The model under review builds one solid part; all positions refer to its coordinate system, in mm. A direction names the side the tool comes from. Give positions to 0.01 mm unless a question says otherwise; leave off trailing zeros. Loops run counter-clockwise (first coordinate to the right, second up) from the corner with the lowest first, then second, coordinate; pieces in that order, holes last. Notation, with made-up numbers: M -14,-32 L -9,-32 A7 ccw -9,-20 Z; hole C -0.75,78.5 d6. An arc over 180 degrees is marked long. Return JSON: item names as keys, results as strings.
```python
from build123d import *

# Parameters (mm, degrees)
F0_W      = 20
F0_H      = 40
F1_DEPTH  = 60
F2_R      = 1.5
F2_R_2    = 10
F3_DEPTH  = 6
F4_R      = 2.25
F5_DEPTH  = 6
F6_R      = 2.25
F7_DEPTH  = 6
F9_R      = 4.5
F9_R_2    = 2.25
F11_DEPTH = 20
F10_R     = 4.5
F10_R_2   = 2.25
F12_DEPTH = 20
F8_R      = 4.5
F8_R_2    = 2.25
F13_DEPTH = 20
F14_DEPTH = 25
F15_DEPTH = 25
F16_DEPTH = 25
F17_DEPTH = 15
F18_DEPTH = 15
F19_DEPTH = 15


with BuildPart() as f1:
    # F0 (on Top) → F1 (new body)
    with BuildSketch(Plane.XY):
        with BuildLine():
            Line((47.3205080757, 53.0098987629), (42.9903810568, 55.5098987629))
            Line((42.9903810568, 55.5098987629), (31.7542648054, 36.0483745358))
            Line((31.7542648054, 36.0483745358), (-31.7542648054, 36.0483745358))
            Line((-31.7542648054, 36.0483745358), (-42.9903810568, 55.5098987629))
            Line((-42.9903810568, 55.5098987629), (-47.3205080757, 53.0098987629))
            Line((-47.3205080757, 53.0098987629), (-17.3205080757, 1.0483745358))
            Line((-17.3205080757, 1.0483745358), (-34.6410161514, -8.9516254642))
            Line((-34.6410161514, -8.9516254642), (-14.6410161514, -43.5926416156))
            ThreePointArc((-14.6410161514, -43.5926416156), (0, -52.0456362318), (14.6410161514, -43.5926416156))
            Line((14.6410161514, -43.5926416156), (34.6410161514, -8.9516254642))
            Line((34.6410161514, -8.9516254642), (17.3205080757, 1.0483745358))
            Line((17.3205080757, 1.0483745358), (47.3205080757, 53.0098987629))
        make_face()
        Polygon((-15, -3.3853821939), (-15, -9.7067520427), (-15, -21.9678594557), (-21.3525872607, -21.9678594557), (-27.8108891325, -10.7817524831), align=None, mode=Mode.SUBTRACT)
        with Locations((0, -18.9516254642)):
            Rectangle(F0_W, F0_H, mode=Mode.SUBTRACT)
        Polygon((15, -21.9678594557), (15, -4.4697315388), (15, -3.3853821939), (27.8108891325, -10.7817524831), (21.3525872607, -21.9678594557), align=None, mode=Mode.SUBTRACT)
        Polygon((28.8675134595, 31.0483745358), (14.4337567297, 6.0483745358), (-14.4337567297, 6.0483745358), (-28.8675134595, 31.0483745358), align=None, mode=Mode.SUBTRACT)
    extrude(amount=F1_DEPTH)

    # F2 (on face) → F3 (cut)
    with BuildSketch(Plane(origin=(0, 36.0483745358, 0), x_dir=(-1, 0, 0), z_dir=(0, 1, 0))):
        with Locations((-15.5, 45.5)):
            Circle(F2_R)
        with Locations((15.5, 45.5)):
            Circle(F2_R)
        with Locations((15.5, 14.5)):
            Circle(F2_R)
        with Locations((-15.5, 14.5)):
            Circle(F2_R)
        with Locations((0, 30)):
            Circle(F2_R_2)
    extrude(amount=-F3_DEPTH, mode=Mode.SUBTRACT)

    # F4 (on face) → F5 (cut)
    with BuildSketch(Plane(origin=(-12.5364215664, -7.237906366, 0), x_dir=(0.5, -0.8660254038, 0), z_dir=(-0.8660254038, -0.5, 0))):
        with Locations((-24.5681730185, 50)):
            Circle(F4_R)
        with Locations((-59.5681730185, 50)):
            Circle(F4_R)
        with Locations((-59.5681730185, 10)):
            Circle(F4_R)
        with Locations((-24.5681730185, 10)):
            Circle(F4_R)
    extrude(amount=-F5_DEPTH, mode=Mode.SUBTRACT)

    # F6 (on face) → F7 (cut)
    with BuildSketch(Plane(origin=(12.5364215664, -7.237906366, 0), x_dir=(0.5, 0.8660254038, 0), z_dir=(0.8660254038, -0.5, 0))):
        with Locations((24.5681730185, 50)):
            Circle(F6_R)
        with Locations((59.5681730185, 50)):
            Circle(F6_R)
        with Locations((59.5681730185, 10)):
            Circle(F6_R)
        with Locations((24.5681730185, 10)):
            Circle(F6_R)
    extrude(amount=-F7_DEPTH, mode=Mode.SUBTRACT)

    # F9 (on face) → F11 (join)
    with BuildSketch(Plane.YZ.offset(-10)):
        with Locations((-28.9516254642, 50)):
            Circle(F9_R)
        with Locations((-28.9516254642, 50)):
            Circle(F9_R_2, mode=Mode.SUBTRACT)
        with Locations((-28.9516254642, 10)):
            Circle(F9_R)
        with Locations((-28.9516254642, 10)):
            Circle(F9_R_2, mode=Mode.SUBTRACT)
    extrude(amount=-F11_DEPTH)

    # F10 (on face) → F12 (join)
    with BuildSketch(Plane(origin=(10, 0, 0), x_dir=(0, -1, 0), z_dir=(-1, 0, 0))):
        with Locations((28.9516254642, 10)):
            Circle(F10_R)
        with Locations((28.9516254642, 10)):
            Circle(F10_R_2, mode=Mode.SUBTRACT)
        with Locations((28.9516254642, 50)):
            Circle(F10_R)
        with Locations((28.9516254642, 50)):
            Circle(F10_R_2, mode=Mode.SUBTRACT)
    extrude(amount=-F12_DEPTH)

    # F8 (on face) → F13 (join)
    with BuildSketch(Plane(origin=(0, -38.9516254642, 0), x_dir=(-1, 0, 0), z_dir=(0, 1, 0))):
        with Locations((0, 50)):
            Circle(F8_R)
        with Locations((0, 50)):
            Circle(F8_R_2, mode=Mode.SUBTRACT)
        with BuildLine():
            ThreePointArc((4.5, 10), (3.1819805153, 13.1819805153), (0, 14.5))
            ThreePointArc((0, 14.5), (-3.1819805153, 6.8180194847), (4.5, 10))
        make_face()
        with BuildLine():
            ThreePointArc((0, 12.25), (1.5909902577, 11.5909902577), (2.25, 10))
            ThreePointArc((2.25, 10), (-1.5909902577, 8.4090097423), (0, 12.25))
        make_face(mode=Mode.SUBTRACT)
    extrude(amount=-F13_DEPTH)

    # F10 (on face) → F14 (cut)
    with BuildSketch(Plane(origin=(10, 0, 0), x_dir=(0, -1, 0), z_dir=(-1, 0, 0))):
        with Locations((28.9516254642, 10)):
            Circle(F10_R_2)
        with Locations((28.9516254642, 50)):
            Circle(F10_R_2)
    extrude(amount=-F14_DEPTH, mode=Mode.SUBTRACT)

    # F9 (on face) → F15 (cut)
    with BuildSketch(Plane.YZ.offset(-10)):
        with Locations((-28.9516254642, 50)):
            Circle(F9_R_2)
        with Locations((-28.9516254642, 10)):
            Circle(F9_R_2)
    extrude(amount=-F15_DEPTH, mode=Mode.SUBTRACT)

    # F8 (on face) → F16 (cut)
    with BuildSketch(Plane(origin=(0, -38.9516254642, 0), x_dir=(-1, 0, 0), z_dir=(0, 1, 0))):
        with Locations((0, 50)):
            Circle(F8_R_2)
        with BuildLine():
            ThreePointArc((0, 12.25), (-1.5909902577, 8.4090097423), (2.25, 10))
            ThreePointArc((2.25, 10), (1.5909902577, 11.5909902577), (0, 12.25))
        make_face()
    extrude(amount=-F16_DEPTH, mode=Mode.SUBTRACT)

    # F17 (cut): faces of the model
    f17_faces = [f1.faces().sort_by_distance(p)[0] for p in [
        (4.3727207794, -58.9516254642, 10),
        (4.3727207794, -58.9516254642, 50),
    ]]
    extrude(f17_faces, amount=-F17_DEPTH, mode=Mode.SUBTRACT)

    # F18 (cut): faces of the model
    f18_faces = [f1.faces().sort_by_distance(p)[0] for p in [
        (30, -24.5789046848, 50),
        (30, -24.5789046848, 10),
    ]]
    extrude(f18_faces, amount=-F18_DEPTH, mode=Mode.SUBTRACT)

    # F19 (cut): faces of the model
    f19_faces = [f1.faces().sort_by_distance(p)[0] for p in [
        (-30, -33.3243462436, 10),
        (-30, -33.3243462436, 50),
    ]]
    extrude(f19_faces, amount=-F19_DEPTH, mode=Mode.SUBTRACT)

    # F22 (on 3pt) → F23 (revolve, cut)
    with BuildSketch(Plane(origin=(-15.0459854695, -0.2184772575, 0), x_dir=(-0.014519104, 0.9998945923, 0), z_dir=(0.9998945923, 0.014519104, 0))):
        Polygon((-3.0741950031, 61.4935897481), (-3.1692667399, 60.0088387728), (31.260818243, 45.5124080181), (31.260818243, 47.0371879637), align=None)
    revolve(axis=Axis((-15.2499175488, 13.8258179605, 52.7606233954), (-0.013381382, 0.9215425078, -0.3880468334)), mode=Mode.SUBTRACT)


solid = f1.part
```
1) Consider section D-D on y = -7.5. Write out the cut boundary in (x, z), then the cut area to 3 significant figures.
From the geometry:
{"outline": "M -32.13,0 L -22.13,0 L -22.13,60 L -32.13,60 Z; M -15,0 L -10,0 L -10,60 L -15,60 Z; M 10,0 L 15,0 L 15,60 L 10,60 Z; M 22.13,0 L 32.13,0 L 32.13,60 L 22.13,60 Z", "area": "1,800 mm²"}
2) Consider section C-C on z = 18. Write out the cut boundary in (x, y), then the cut area to 3 significant figures.
From the geometry:
{"outline": "M -47.32,53.01 L -17.32,1.05 L -34.64,-8.95 L -14.64,-43.59 A16.91 ccw 14.64,-43.59 L 34.64,-8.95 L 17.32,1.05 L 47.32,53.01 L 42.99,55.51 L 31.75,36.05 L -31.75,36.05 L -42.99,55.51 Z; hole M -28.87,31.05 L -14.43,6.05 L 14.43,6.05 L 28.87,31.05 Z; hole M -27.81,-10.78 L -21.35,-21.97 L -15,-21.97 L -15,-3.39 Z; hole M -10,-38.95 L 10,-38.95 L 10,1.05 L -10,1.05 Z; hole M 15,-21.97 L 21.35,-21.97 L 27.81,-10.78 L 15,-3.39 Z", "area": "2,340 mm²"}
3) The part is to be moulded in two halves that separate along Z. For faces 5 (the face through (-15, -13, 30)), 6 (the face through (0.29, -41.42, 52.23)), say which applies: released by +Z, released by -Z, zero draft, split by the parting line, or undercut.
From the geometry:
{"face 5": "zero draft", "face 6": "undercut"}
4) Insertion check: pin 1 (7 mm diameter, centred on y = -28.95, z = 50, fed in from -X); pin 2 (5 mm diameter, centred on x = 29, z = 28.5, fed in from +Y); pin 3 (5.5 mm diameter, centred on x = 0, z = 10, fed in from -Y); pin 4 (2.5 mm diameter, centred on y = -28.95, z = 50, fed in from -X). Each pin has a flat end and moves straight along its axis. Give the tip position at first contact, or say it passes through.
From the geometry:
{"pin 1": "x = -15", "pin 2": "y = 36.05", "pin 3": "y = -43.95", "pin 4": "through"}
5) Consider section A-A on z = 30. Count the separate pieces of the cut face and the enclosed holes in it, then the cut area to 3 significant figures.
From the geometry:
{"separate pieces": "1", "enclosed holes": "3", "area": "2,240 mm²"}
6) Tool access review of faces 1 (the face through (15, -31, 8)), 2 (the face through (-15, -27, 48)), 3 (the face through (-14, 33.58, 14.57)), 4 (the face through (4.496, -48.055, 50.198)): name each direction out of +Z, -Z, +X, -X, +Y, -Y from which nothing blocks a thin tool from reaching the whole face with its end or side.
From the geometry:
{"face 1": "+X", "face 2": "-X", "face 3": "+Y", "face 4": "-Y"}
7) Consider section B-B on x = -7. Write out the cut boundary in (y, z).
From the geometry:
{"outline": "M -50.53,0 L -38.95,0 L -38.95,60 L -50.53,60 Z; M 1.05,0 L 6.05,0 L 6.05,60 L 1.05,60 Z; M 31.05,0 L 36.05,0 L 36.05,22.86 L 31.05,22.86 Z; M 31.05,37.14 L 36.05,37.14 L 36.05,60 L 31.05,60 Z"}
8) Wall thickness on L1, parallel to Z at x = 0, y = -49; L2, parallel to Y at x = 0.5, z = 18; L3, parallel to Z at x = 0, y = -42.25: over which ranges is each line inside the solid? List them lowest first. Write a range as from..to.
From the geometry:
{"L1": "0..5.5, 14.5..45.5, 54.5..60", "L2": "-52.04..-38.95, 1.05..6.05, 31.05..36.05", "L3": "0..7.75, 12.25..47.75, 52.25..60"}
